Model file for the job. Use its own axes, mm. Face numbers are marked on the shaded views. A direction names the side the tool comes from. Round coordinates to 2 decimals unless told otherwise and drop trailing zeros. Loops run counter-clockwise (first coordinate to the right, second up) from the corner with the lowest first, then second, coordinate; pieces in that order, holes last. Notation, with made-up numbers: M -2.5,71 L 37.5,71 A24 ccw 37.5,105 Z; hole C 64.5,-38 d7. An arc over 180 degrees is marked long. Use a Markdown table: item, result. Add a question column.
Item 1: Saw through at B-B on x = 0. Write the cut outline in (y, z), then the cut area to 3 significant figures.
Item 2: Wall check: L1, parallel to Y at x = 0, z = 0.6; L2, parallel to Z at x = 7.75, y = 7; L3, parallel to X at y = 2.5, z = 7.5. Give the ranges that are in metal, low to high. Write a range as from..to.
Item 3: Tool access for the marked faces 5, 6, 7, 8 and 9: list every direction of +Z, -Z, +X, -X, +Y, -Y with a clear straight run to the whole face (end or side of a thin tool).
Item 4: Saw through at A-A on y = 0. Write the cut outline in (x, z).
Item 5: Saw through at D-D on z = 2.5. Write the cut outline in (x, y), then the cut area to 3 significant figures.
Item 6: Saw through at C-C on y = 10.75. Write the cut outline in (x, z), then the cut area to 3 significant figures.
Item 7: Pin check, flat tips, straight feed: P1, Ø3.5, axis at x = 8.56, y = -4.94, coming from the +Z side; P2, Ø2.5, axis at y = -1, z = 8, coming from the +X side; P3, Ø4, axis at y = 1.5, z = 5.5, coming from the -X side; P4, Ø6, axis at y = 3, z = 3.5, coming from the -X side. Stop position of each tip, or through.
Item 8: Two-plate mould, pull along X, no slides. Class the marked faces 1, 2, 3 and 4: +X half, -X half, draft (parallel to the pull), parting line (faces both ways), or undercut.
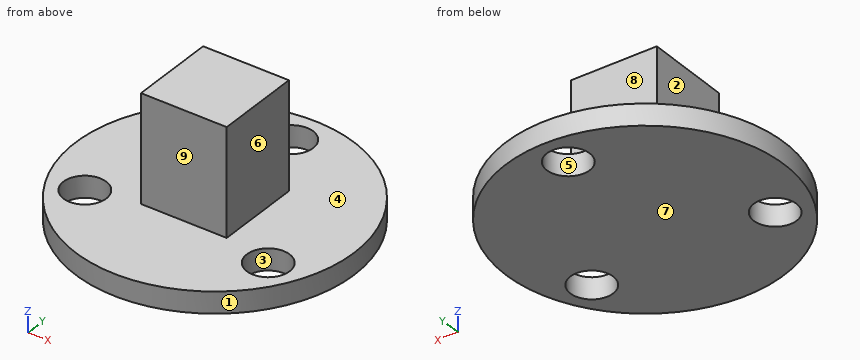
```python
from build123d import *

# Parameters (mm, degrees)
F0_R     = 13
F1_DEPTH = 2
F2_W     = 8
F2_H     = 8
F3_DEPTH = 10
F4_R     = 2
F5_DEPTH = 25


with BuildPart() as f1:
    # F0 (on Top) → F1 (new body)
    with BuildSketch(Plane.XY):
        Circle(F0_R)
    extrude(amount=F1_DEPTH)

    # F2 (on face) → F3 (join)
    with BuildSketch(Plane.XY.offset(2)):
        Rectangle(F2_W, F2_H)
    extrude(amount=F3_DEPTH)

    # F4 (on face) → F5 (cut)
    with BuildSketch(Plane.XY.offset(2)):
        with Locations((0, 9.881104)):
            Circle(F4_R)
        with Locations((8.557287, -4.940552)):
            Circle(F4_R)
        with Locations((-8.557287, -4.940552)):
            Circle(F4_R)
    extrude(amount=-F5_DEPTH, mode=Mode.SUBTRACT)


solid = f1.part
```
Entries:
| question | item | result |
|---|---|---|
| 1 | outline | M -13,0 L 7.88,0 L 7.88,2 L 4,2 L 4,12 L -4,12 L -4,2 L -13,2 Z; M 11.88,0 L 13,0 L 13,2 L 11.88,2 Z |
| 1 | area | 124 mm2 |
| 2 | L1 | -13..7.88, 11.88..13 |
| 2 | L2 | 0..2 |
| 2 | L3 | -4..4 |
| 3 | face 5 | +Z, -Z |
| 3 | face 6 | +Z, +X, +Y, -Y |
| 3 | face 7 | -Z, +X, -X, +Y, -Y |
| 3 | face 8 | +Z, +X, -X, +Y |
| 3 | face 9 | +Z, +X, -X, -Y |
| 4 | outline | M -13,0 L 13,0 L 13,2 L 4,2 L 4,12 L -4,12 L -4,2 L -13,2 Z |
| 5 | outline | M -4,-4 L 4,-4 L 4,4 L -4,4 Z |
| 5 | area | 64.0 mm2 |
| 6 | outline | M -7.31,0 L -1.8,0 L -1.8,2 L -7.31,2 Z; M 1.8,0 L 7.31,0 L 7.31,2 L 1.8,2 Z |
| 6 | area | 22.0 mm2 |
| 7 | P1 | through |
| 7 | P2 | x = 4 |
| 7 | P3 | x = -4 |
| 7 | P4 | x = -12.99 |
| 8 | face 1 | parting line |
| 8 | face 2 | -X half |
| 8 | face 3 | undercut |
| 8 | face 4 | draft |
